Design review of the part shown in the three views and the two pictorial views. Dimensions are in mm from the part's minimum x, y and z. Give positions to 0.01 mm unless a question says otherwise; leave off trailing zeros. Write each loop counter-clockwise with the first axis right and the second up, starting at its lowest first coordinate (ties: lowest second). Pieces come first, ordered by that corner, then holes.
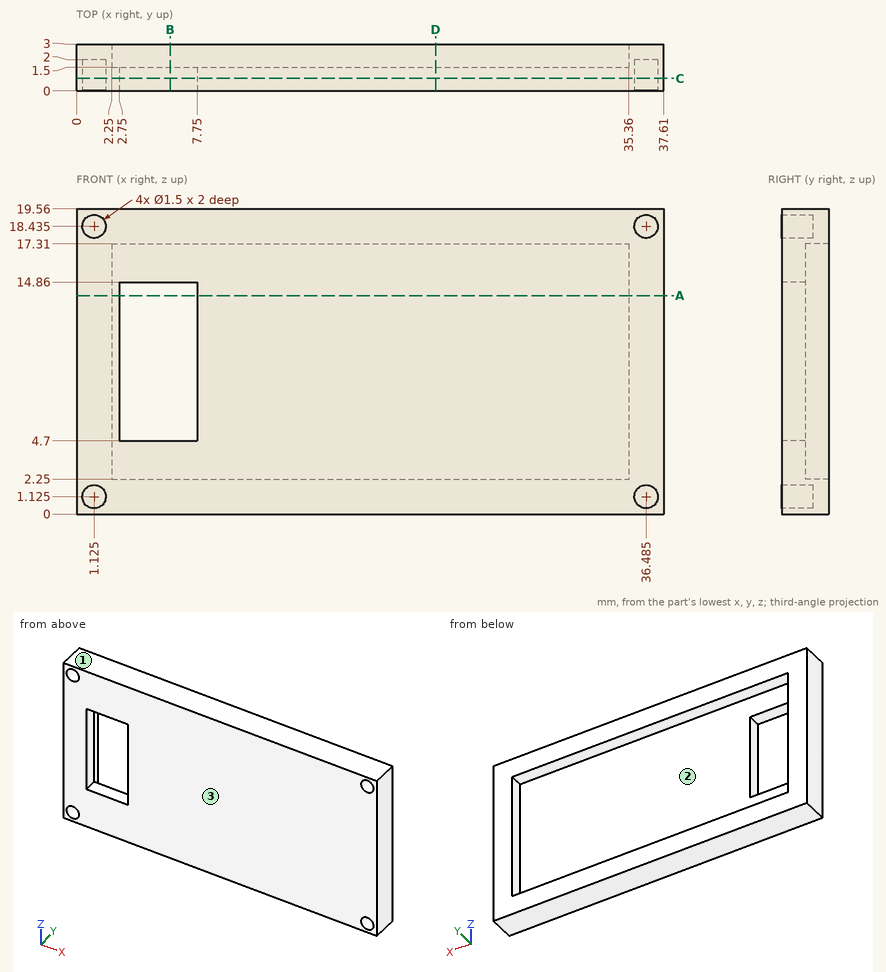
(1) Mouldability with a two-part tool opening along Z and no side actions: class the marked faces 1, 2 and 3 as pulls with the +Z half, pulls with the -Z half, needs draft (parallel to the pull), parting line crosses it, or undercut.
Resolved:
face 1: pulls with the +Z half
face 2: undercut
face 3: needs draft
(2) Consider section B-B, the plane x = 6. Give the boundary of the cut face in (y, z), then the cut area to 4 significant figures.
Resolved:
outline: (0, 0) - (3, 0) - (3, 2.25) - (1.5, 2.25) - (1.5, 4.7) - (0, 4.7) - close; (0, 14.86) - (1.5, 14.86) - (1.5, 17.31) - (3, 17.31) - (3, 19.56) - (0, 19.56) - close
area: 20.85 mm2
(3) To check wall thickness, follow L1, parallel to Z at x = 23.5, y = 2.15; L2, parallel to X at y = 2.1, z = 14.5; L3, parallel to X at y = 1.3, z = 6.5. State the ranges of each line that lie inside material, in increasing order.
Resolved:
L1: z = 0 to 2.25, 17.31 to 19.56
L2: x = 0 to 2.25, 35.36 to 37.61
L3: x = 0 to 2.75, 7.75 to 37.61
(4) Clearance check with flat-ended pins moving along their axes: P1, Ø1.2, axis at y = 2.5, z = 11, coming from the -X side; P2, Ø4.5, axis at x = 26, z = 9.5, coming from the +Y side; P3, Ø1.2, axis at x = 36.5, z = 18.5, coming from the -Y side. State where each tip first meets the part, or that it passes through.
Resolved:
P1: stops at x = 0
P2: stops at y = 1.5
P3: stops at y = 2
(5) Consider section C-C, the plane y = 0.8. Give the boundary of the cut face in (x, z) (3 decimals).
Resolved:
outline: (0, 0) - (37.61, 0) - (37.61, 19.56) - (0, 19.56) - close; hole circle Ø1.5 at (1.125, 1.125); hole circle Ø1.5 at (1.125, 18.435); hole (2.75, 4.7) - (7.75, 4.7) - (7.75, 14.86) - (2.75, 14.86) - close; hole circle Ø1.5 at (36.485, 1.125); hole circle Ø1.5 at (36.485, 18.435)
(6) Consider section D-D, the plane x = 23. Give the boundary of the cut face in (y, z), then the cut area to 3 significant figures.
Resolved:
outline: (0, 0) - (3, 0) - (3, 2.25) - (1.5, 2.25) - (1.5, 17.31) - (3, 17.31) - (3, 19.56) - (0, 19.56) - close
area: 36.1 mm2
(7) Consider section A-A, the plane z = 14. Give the boundary of the cut face in (x, y), then the cut area to 3 significant figures.
Resolved:
outline: (0, 0) - (2.75, 0) - (2.75, 1.5) - (2.25, 1.5) - (2.25, 3) - (0, 3) - close; (7.75, 0) - (37.61, 0) - (37.61, 3) - (35.36, 3) - (35.36, 1.5) - (7.75, 1.5) - close
area: 55.7 mm2
